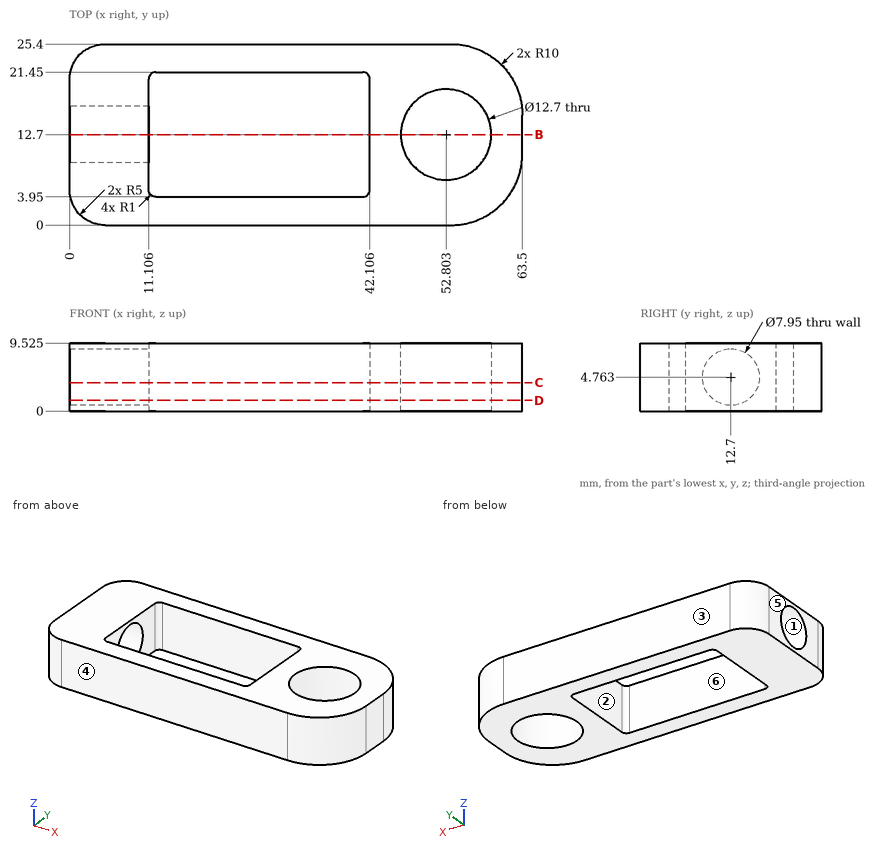
Geometry check sheet. Reference: drawing and pictorial views, mm from the part's lowest x, y, z. A direction names the side the tool comes from. Round coordinates to 2 decimals unless told otherwise and drop trailing zeros. Loops run counter-clockwise (first coordinate to the right, second up) from the corner with the lowest first, then second, coordinate; pieces in that order, holes last.
1. Gauge pin test, flat ends, axial feed: pin 1 Ø8 at (x, y) = (49, 19) entering from -Z; pin 2 Ø1 at (y, z) = (12.5, 2) entering from -X. Record the tip position at first contact, or that the pin passes through.
2. Scan lines: probe 1 along Y at (x, z) = (26.5, 1.5); probe 2 along X at (y, z) = (12.75, 5.5); probe 3 along X at (y, z) = (19.5, 4.5) (1 decimal). Record each from-to range of solid material in increasing order.
3. Mould release check, pull along X, two halves, no side actions. Record for the marked faces 4, 5 and 6: released by +X, released by -X, zero draft, split by the parting line, or undercut.
4. Sectioned sample at C-C on z = 4. Record the boundary of the cut face in (x, y).
5. Sectioned sample at D-D on z = 1.5. Record the boundary of the cut face in (x, y).
6. Set-up check for the marked faces 1, 2 and 3: record each of +Z, -Z, +X, -X, +Y, -Y from which the full face is reachable in a straight line by a thin tool's end or side.
7. Sectioned sample at B-B on y = 12.7. Record the boundary of the cut face in (x, z) (1 decimal).
Recorded:
1. pin 1: stops at z = 0
1. pin 2: stops at x = 42.11
2. probe 1: y = 0 to 3.95, 21.45 to 25.4
2. probe 2: x = 42.11 to 46.45, 59.15 to 63.5
2. probe 3: x = 0 to 11.1, 42.1 to 62.6
3. face 4: zero draft
3. face 5: released by -X
3. face 6: undercut
4. outline: (0, 5) arc R5 ccw to (5, 0) - (53.5, 0) arc R10 ccw to (63.5, 10) - (63.5, 15.4) arc R10 ccw to (53.5, 25.4) - (5, 25.4) arc R5 ccw to (0, 20.4) - (0, 16.6) - (11.11, 16.6) - (11.11, 20.45) arc R1 cw to (12.11, 21.45) - (41.11, 21.45) arc R1 cw to (42.11, 20.45) - (42.11, 4.95) arc R1 cw to (41.11, 3.95) - (12.11, 3.95) arc R1 cw to (11.11, 4.95) - (11.11, 8.8) - (0, 8.8) - close; hole circle Ø12.7 at (52.8, 12.7)
5. outline: (0, 5) arc R5 ccw to (5, 0) - (53.5, 0) arc R10 ccw to (63.5, 10) - (63.5, 15.4) arc R10 ccw to (53.5, 25.4) - (5, 25.4) arc R5 ccw to (0, 20.4) - (0, 14.97) - (11.11, 14.97) - (11.11, 20.45) arc R1 cw to (12.11, 21.45) - (41.11, 21.45) arc R1 cw to (42.11, 20.45) - (42.11, 4.95) arc R1 cw to (41.11, 3.95) - (12.11, 3.95) arc R1 cw to (11.11, 4.95) - (11.11, 10.43) - (0, 10.43) - close; hole circle Ø12.7 at (52.8, 12.7)
6. face 1: -X
6. face 2: +Z, -Z
6. face 3: +Z, -Z, +X, -X, +Y
7. outline: (0, 0) - (11.1, 0) - (11.1, 0.8) - (0, 0.8) - close; (0, 8.7) - (11.1, 8.7) - (11.1, 9.5) - (0, 9.5) - close; (42.1, 0) - (46.5, 0) - (46.5, 9.5) - (42.1, 9.5) - close; (59.2, 0) - (63.5, 0) - (63.5, 9.5) - (59.2, 9.5) - close
